from build123d import *

# Parameters (mm, degrees)
PAD_DEPTH         = 0.25
PAD001_DEPTH      = 1.1
PAD001_DEPTH_BACK = 2.3


with BuildPart() as pad:
    # Sketch → Pad (new body, symmetric)
    with BuildSketch(Plane.XZ):
        Polygon((-2.04, 2), (-2.04, 0), (-0.5, 0), (-0.5, -15), (0, -16), (0.5, -15), (0.5, 2), align=None)
        Polygon((14.74, 2), (14.74, -15), (15.24, -16), (15.74, -15), (15.74, 0), (17.28, 0), (17.28, 2), align=None)
        Polygon((4.08, 2), (4.08, 0), (4.58, 0), (4.58, -15), (5.08, -16), (5.58, -15), (5.58, 0), (6.08, 0), (6.08, 2), align=None)
        Polygon((9.16, 2), (9.16, -0.056881), (9.66, -0.056881), (9.66, -15), (10.16, -16), (10.66, -15), (10.66, -0.056881), (11.16, -0.056881), (11.16, 2), align=None)
    extrude(amount=PAD_DEPTH, both=True)


with BuildPart() as obj1:
    # Sketch001 → Pad001 (new body, two sides)
    with BuildSketch(Plane(origin=(15.24, 0, 0), x_dir=(-1, 0, 0), z_dir=(0, 1, 0))) as pad001_sk:
        with BuildLine():
            Line((-2.43, 1.9), (17.67, 1.9))
            ThreePointArc((17.67, 1.9), (18.377107, 2.192893), (18.67, 2.9))
            Line((18.67, 2.9), (18.67, 17.2))
            Line((18.67, 17.2), (15.47, 20.4))
            Line((15.47, 20.4), (-2.43, 20.4))
            ThreePointArc((-2.43, 20.4), (-3.137107, 20.107107), (-3.43, 19.4))
            Line((-3.43, 19.4), (-3.43, 2.9))
            ThreePointArc((-3.43, 2.9), (-3.137107, 2.192893), (-2.43, 1.9))
        make_face()
        with BuildLine():
            ThreePointArc((9.52, 12.8), (7.62, 14.7), (5.72, 12.8))
            Line((5.72, 12.8), (5.72, 10.95))
            ThreePointArc((5.72, 10.95), (7.62, 9.05), (9.52, 10.95))
            Line((9.52, 12.8), (9.52, 10.95))
        make_face(mode=Mode.SUBTRACT)
    extrude(amount=PAD001_DEPTH)
    extrude(pad001_sk.sketch, amount=-PAD001_DEPTH_BACK)

    add(pad.part)


solid = obj1.part
Can you work these out from the model? Positions are in its coordinate system, mm. A direction names the side the tool comes from. Give positions to 0.01 mm unless a question says otherwise; leave off trailing zeros. Loops run counter-clockwise (first coordinate to the right, second up) from the corner with the lowest first, then second, coordinate; pieces in that order, holes last. Notation, with made-up numbers: M 28.5,21 L 46.5,21 A28 cw 46.5,41 Z; hole C -16.5,-10.5 d11. An arc over 180 degrees is marked long. One line per item, written item: value.
1) Thinking about a two-plate mould opening in Z: for faces 1 (the face through (9.52, -1, 12)), 2 (the face through (7.66, -0.58, 9.05)), 3 (the face through (15, 0.25, -7)), 4 (the face through (9, -1, 20.4)), which applies, +Z half, -Z half, draft (parallel to the pull), parting line (faces both ways), or undercut?
Geometry check:
face 1: undercut
face 2: undercut
face 3: draft
face 4: +Z half
2) Please list where these lines run through material, in increasing order: line 1 (X direction, y = 0.2, z = -10.5); line 2 (Z direction, x = 1.25, y = -0.05); line 3 (X direction, y = -0.65, z = 14).
Geometry check:
line 1: x = -0.5 to 0.5, 4.58 to 5.58, 9.66 to 10.66, 14.74 to 15.74
line 2: z = 1.9 to 20.4
line 3: x = -3.43 to 6.15, 9.09 to 18.67
3) Imagine slicing it at A-A on y = -1.25. Write out the boundary of the cut face in (x, z).
Geometry check:
outline: M -3.43,2.9 A1 ccw -2.43,1.9 L 17.67,1.9 A1 ccw 18.67,2.9 L 18.67,19.4 A1 ccw 17.67,20.4 L -0.23,20.4 L -3.43,17.2 Z; hole M 5.72,10.95 A1.9 ccw 9.52,10.95 L 9.52,12.8 A1.9 ccw 5.72,12.8 Z
4) I'm going to push flat-ended pins straight in: pin 1 (0.6 mm diameter, centred on x = 11, y = 0, fed in from -Z); pin 2 (3 mm diameter, centred on x = -1, z = -4, fed in from +Y); pin 3 (1.3 mm diameter, centred on x = 15.5, z = -6.5, fed in from -Y). Where does each tip first touch, or does it pass through?
Geometry check:
pin 1: stops at z = -0.06
pin 2: stops at y = 0.25
pin 3: stops at y = -0.25
5) Imagine slicing it at B-B on z = -3. Write out the boundary of the cut face in (x, y), and give its area (3 significant figures).
Geometry check:
outline: M -0.5,-0.25 L 0.5,-0.25 L 0.5,0.25 L -0.5,0.25 Z; M 4.58,-0.25 L 5.58,-0.25 L 5.58,0.25 L 4.58,0.25 Z; M 9.66,-0.25 L 10.66,-0.25 L 10.66,0.25 L 9.66,0.25 Z; M 14.74,-0.25 L 15.74,-0.25 L 15.74,0.25 L 14.74,0.25 Z
area: 2.00 mm²
6) Imagine slicing it at C-C on x = 7.62. Write out the boundary of the cut face in (y, z).
Geometry check:
outline: M -2.3,1.9 L 1.1,1.9 L 1.1,9.05 L -2.3,9.05 Z; M -2.3,14.7 L 1.1,14.7 L 1.1,20.4 L -2.3,20.4 Z
7) On a 3-axis mill with a long thin cutter (end or side, diameter ignored), from which of +Z, -Z, +X, -X, +Y, -Y can I reach the whole of each face in a straight line? I mean faces 5 (the face through (10, -0.25, -7)), 6 (the face through (18.369, -0.576, 20.115)), 7 (the face through (0, 0.25, -5)), 8 (the face through (18.385, -0.576, 2.201)), 9 (the face through (5.72, -1, 12)). Say none if no direction works.
Geometry check:
face 5: -Z, +X, -X, -Y
face 6: +Z, +X, +Y, -Y
face 7: -Z, +X, -X, +Y
face 8: -Z, +X, +Y, -Y
face 9: +Y, -Y
